Verification items for the finished model (mm, model axes). Face numbers are marked on the shaded views. A direction names the side the tool comes from. Round coordinates to 2 decimals unless told otherwise and drop trailing zeros. Loops run counter-clockwise (first coordinate to the right, second up) from the corner with the lowest first, then second, coordinate; pieces in that order, holes last. Notation, with made-up numbers: (31, -40) -> (84, -40) arc R23 cw to (84, -16) -> close; hole circle Ø7 at (-8.75, 85). An arc over 180 degrees is marked (long way). Write item = value, one per line. Start each with the question number.
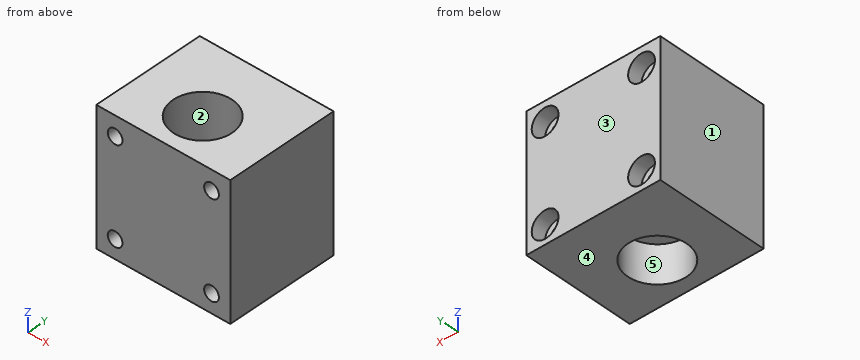
```python
from build123d import *

# Parameters (mm, degrees)
EXTRUDE_608_DEPTH          = 50
SKETCH_2_R                 = 11
CUT_EXTRUDE_1_DEPTH        = 14
CUT_EXTRUDE_START          = -30
SKETCH_3_R                 = 11
CUT_EXTRUDE_2_DEPTH        = 30
SKETCH_4_R                 = 6.5
CUT_EXTRUDE_3_DEPTH        = 60.715994507
HOLE_WIZARD_M5_D           = 5.5
HOLE_WIZARD_M5_CBORE_D     = 10
HOLE_WIZARD_M5_CBORE_DEPTH = 5.4


with BuildPart() as part:
    # Эскиз1 → Extrude 608 (new body)
    with BuildSketch(Plane.XY):
        Polygon((-25, 21), (0, 21), (25, 21), (25, -21), (-25, -21), align=None)
    extrude(amount=-EXTRUDE_608_DEPTH)

    # Эскиз2 → Вырез-Вытянуть1 (cut)
    with BuildSketch(Plane(origin=(0, 0, -50), x_dir=(-1, 0, 0), z_dir=(0, 0, -1))):
        with Locations((0, -5)):
            Circle(SKETCH_2_R)
    extrude(amount=-CUT_EXTRUDE_1_DEPTH, mode=Mode.SUBTRACT)

    # Эскиз3 → Вырез-Вытянуть2 (cut)
    with BuildSketch(Plane.XY.offset(CUT_EXTRUDE_START)):
        with Locations(Location((0, -5, 0), (0, 0, 180))):
            Circle(SKETCH_3_R)
    extrude(amount=CUT_EXTRUDE_2_DEPTH, mode=Mode.SUBTRACT)

    # Эскиз4 → Вырез-Вытянуть3 (cut, through all)
    with BuildSketch(Plane.XY):
        with Locations((0, -5)):
            Circle(SKETCH_4_R)
    extrude(amount=-CUT_EXTRUDE_3_DEPTH, mode=Mode.SUBTRACT)

    # Крепление M5 (through all)
    with Locations(Plane(origin=(0, 21, 0), x_dir=(1, 0, 0), z_dir=(0, 1, 0))):
        with Locations((-18, 43), (-18, 7.344841497), (18, 7.344841497), (18, 43)):
            CounterBoreHole(HOLE_WIZARD_M5_D / 2, HOLE_WIZARD_M5_CBORE_D / 2, HOLE_WIZARD_M5_CBORE_DEPTH)


solid = part.part
```
(1) Depth check by flat-ended pin: pin 1 Ø9 at (x, z) = (-18, -7.34) entering from +Y; pin 2 Ø4.5 at (x, z) = (18, -43) entering from +Y; pin 3 Ø17.5 at (x, y) = (0, -5) entering from -Z. Enter the tip coordinate at first touch or a pass-through.
(2) Scan lines: line 1 (Z direction, x = -18, y = -3.5); line 2 (Z direction, x = 18, y = 17.8); line 3 (Y direction, x = 0.5, z = -23). Record each from-to range of solid material in increasing order. Write a range as [from, to].
(3) Access from +Z, -Z, +X, -X, +Y, -Y to the whole of each face (thin tool, end or side, straight path). Record for the marked faces 4 and 5.
(4) Section check A-A on z = -43. Enter the section's corners in (x, y), then the cut area to 3 significant figures.
(5) Section check C-C on x = -18. Enter the section's corners in (y, z).
(6) Section check D-D on x = 0. Enter the section's corners in (y, z).
(7) Draft check along X on the marked faces 1, 2 and 3. Enter one of: +X half, -X half, draft (parallel to the pull), parting line (faces both ways), or undercut.
(8) Section check B-B on y = -10.5. Enter the section's corners in (x, z).
Computed values:
q1.pin_1 = 15.6
q1.pin_2 = through
q1.pin_3 = -36
q2.line_1 = [-50, -45.75], [-40.25, -10.09], [-4.59, 0]
q2.line_2 = [-50, -48], [-38, -12.34], [-2.34, 0]
q2.line_3 = [-21, -15.99], [5.99, 21]
q3.face_4 = -Z, +X, -X, +Y, -Y
q3.face_5 = -Z
q4.outline = (-25, -21) -> (-20.75, -21) -> (-20.75, 15.6) -> (-23, 15.6) -> (-23, 21) -> (-25, 21) -> close; (-15.25, -21) -> (15.25, -21) -> (15.25, 15.6) -> (13, 15.6) -> (13, 21) -> (-13, 21) -> (-13, 15.6) -> (-15.25, 15.6) -> close; (20.75, -21) -> (25, -21) -> (25, 21) -> (23, 21) -> (23, 15.6) -> (20.75, 15.6) -> close; hole circle Ø22 at (0, -5)
q4.area = 1,210 mm²
q5.outline = (-21, -50) -> (21, -50) -> (21, -48) -> (15.6, -48) -> (15.6, -45.75) -> (-21, -45.75) -> close; (-21, -40.25) -> (15.6, -40.25) -> (15.6, -38) -> (21, -38) -> (21, -12.34) -> (15.6, -12.34) -> (15.6, -10.09) -> (-21, -10.09) -> close; (-21, -4.59) -> (15.6, -4.59) -> (15.6, -2.34) -> (21, -2.34) -> (21, 0) -> (-21, 0) -> close
q6.outline = (-21, -50) -> (-16, -50) -> (-16, -36) -> (-11.5, -36) -> (-11.5, -30) -> (-16, -30) -> (-16, 0) -> (-21, 0) -> close; (1.5, -36) -> (6, -36) -> (6, -50) -> (21, -50) -> (21, 0) -> (6, 0) -> (6, -30) -> (1.5, -30) -> close
q7.face_1 = -X half
q7.face_2 = undercut
q7.face_3 = draft
q8.outline = (-25, -50) -> (-9.53, -50) -> (-9.53, -36) -> (-3.46, -36) -> (-3.46, -30) -> (-9.53, -30) -> (-9.53, 0) -> (-25, 0) -> close; (3.46, -36) -> (9.53, -36) -> (9.53, -50) -> (25, -50) -> (25, 0) -> (9.53, 0) -> (9.53, -30) -> (3.46, -30) -> close; hole circle Ø5.5 at (-18, -43); hole circle Ø5.5 at (-18, -7.34); hole circle Ø5.5 at (18, -43); hole circle Ø5.5 at (18, -7.34)
